Check sheet for the modelled part. Datum: model origin and axes. Units: mm. A direction names the side the tool comes from. Round coordinates to 2 decimals unless told otherwise and drop trailing zeros. Order: outer loops, then holes, each group sorted by start corner. A loop starts at its lowest first (then second) coordinate and runs counter-clockwise, first axis right, second up.
from build123d import *

# Parameters (mm, degrees)
BOSS_EXTRUDE1_DEPTH           = 4
BOSS_EXTRUDE1_DRAFT           = -2
SHELL1_T                      = -0.5
BOSS_EXTRUDE2_DEPTH           = 5.5
BOSS_EXTRUDE2_DRAFT           = 1.5
BOSS_EXTRUDE2_PROFILE_2_DEPTH = 5.5
BOSS_EXTRUDE2_PROFILE_2_DRAFT = 1.5
BOSS_EXTRUDE2_PROFILE_3_DEPTH = 5.5
BOSS_EXTRUDE2_PROFILE_3_DRAFT = 1.5
BOSS_EXTRUDE2_PROFILE_4_DEPTH = 5.5
BOSS_EXTRUDE2_PROFILE_4_DRAFT = 1.5


with BuildPart() as part:
    # Sketch1 → Boss-Extrude1 (with draft: the straight prism first)
    with BuildSketch(Plane(origin=(0, 0, 0), x_dir=(1, 0, 0), z_dir=(0, 1, 0))):
        with BuildLine():
            Line((-7.5, -6.375), (7.5, -6.375))
            ThreePointArc((7.5, -6.375), (8.207106781, -6.082106781), (8.5, -5.375))
            Line((8.5, -5.375), (8.5, 5.375))
            ThreePointArc((8.5, 5.375), (8.207106781, 6.082106781), (7.5, 6.375))
            Line((7.5, 6.375), (-7.5, 6.375))
            ThreePointArc((-7.5, 6.375), (-8.207106781, 6.082106781), (-8.5, 5.375))
            Line((-8.5, 5.375), (-8.5, -5.375))
            ThreePointArc((-8.5, -5.375), (-8.207106781, -6.082106781), (-7.5, -6.375))
        make_face()
    extrude(amount=-BOSS_EXTRUDE1_DEPTH)
    # Boss-Extrude1: the draft: its side faces are tilted about the plane it starts from
    boss_extrude1_sides = [part.faces().sort_by_distance(p)[0] for p in [
        (0, -2, 6.375),
        (8.207106781, -2, 6.082106781),
        (8.5, -2, 0),
        (8.207106781, -2, -6.082106781),
        (0, -2, -6.375),
        (-8.207106781, -2, -6.082106781),
        (-8.5, -2, 0),
        (-8.207106781, -2, 6.082106781),
    ]]
    draft(boss_extrude1_sides, Plane(origin=(0, 0, 0), x_dir=(1, 0, 0), z_dir=(0, 1, 0)), BOSS_EXTRUDE1_DRAFT)

    # Shell1
    shell1_openings = [part.faces().sort_by_distance(p)[0] for p in [
        (0, 0, 0),
    ]]
    offset(amount=SHELL1_T, openings=shell1_openings, kind=Kind.INTERSECTION)


with BuildPart() as boss_extrude2_tool:
    # Sketch3 → Boss-Extrude2 (with draft: the straight prism first)
    with BuildSketch(Plane(origin=(0, -3.5, 0), x_dir=(1, 0, 0), z_dir=(0, 1, 0))):
        with BuildLine():
            ThreePointArc((-0.6, 2.897704648), (-2.092449787, 2.092449787), (-2.897704648, 0.6))
            Line((-2.897704648, 0.6), (-0.6, 0.6))
            Line((-0.6, 0.6), (-0.6, 2.897704648))
        make_face()
    extrude(amount=BOSS_EXTRUDE2_DEPTH)
    # Boss-Extrude2: the draft: its side faces are tilted about the plane it starts from
    boss_extrude2_sides = [boss_extrude2_tool.faces().sort_by_distance(p)[0] for p in [
        (-2.092449787, -0.75, -2.092449787),
        (-1.748852324, -0.75, -0.6),
        (-0.6, -0.75, -1.748852324),
    ]]
    draft(boss_extrude2_sides, Plane(origin=(0, -3.5, 0), x_dir=(1, 0, 0), z_dir=(0, 1, 0)), BOSS_EXTRUDE2_DRAFT)


with BuildPart() as part_1:
    add(part.part)

    # Boss-Extrude2: add boss_extrude2_tool
    add(boss_extrude2_tool.part)


with BuildPart() as boss_extrude2_profile_2_tool:
    # Sketch3 → Boss-Extrude2 profile 2 (with draft: the straight prism first)
    with BuildSketch(Plane(origin=(0, -3.5, 0), x_dir=(1, 0, 0), z_dir=(0, 1, 0))):
        with BuildLine():
            Line((0.6, 2.897704648), (0.6, 0.6))
            Line((0.6, 0.6), (2.897704648, 0.6))
            ThreePointArc((2.897704648, 0.6), (2.092449787, 2.092449787), (0.6, 2.897704648))
        make_face()
    extrude(amount=BOSS_EXTRUDE2_PROFILE_2_DEPTH)
    # Boss-Extrude2 profile 2: the draft: its side faces are tilted about the plane it starts from
    boss_extrude2_profile_2_sides = [boss_extrude2_profile_2_tool.faces().sort_by_distance(p)[0] for p in [
        (2.092449787, -0.75, -2.092449787),
        (0.6, -0.75, -1.748852324),
        (1.748852324, -0.75, -0.6),
    ]]
    draft(boss_extrude2_profile_2_sides, Plane(origin=(0, -3.5, 0), x_dir=(1, 0, 0), z_dir=(0, 1, 0)), BOSS_EXTRUDE2_PROFILE_2_DRAFT)


with BuildPart() as part_2:
    add(part_1.part)

    # Boss-Extrude2 profile 2: add boss_extrude2_profile_2_tool
    add(boss_extrude2_profile_2_tool.part)


with BuildPart() as boss_extrude2_profile_3_tool:
    # Sketch3 → Boss-Extrude2 profile 3 (with draft: the straight prism first)
    with BuildSketch(Plane(origin=(0, -3.5, 0), x_dir=(1, 0, 0), z_dir=(0, 1, 0))):
        with BuildLine():
            ThreePointArc((-2.897704648, -0.6), (-2.092449787, -2.092449787), (-0.6, -2.897704648))
            Line((-0.6, -2.897704648), (-0.6, -0.6))
            Line((-0.6, -0.6), (-2.897704648, -0.6))
        make_face()
    extrude(amount=BOSS_EXTRUDE2_PROFILE_3_DEPTH)
    # Boss-Extrude2 profile 3: the draft: its side faces are tilted about the plane it starts from
    boss_extrude2_profile_3_sides = [boss_extrude2_profile_3_tool.faces().sort_by_distance(p)[0] for p in [
        (-2.092449787, -0.75, 2.092449787),
        (-0.6, -0.75, 1.748852324),
        (-1.748852324, -0.75, 0.6),
    ]]
    draft(boss_extrude2_profile_3_sides, Plane(origin=(0, -3.5, 0), x_dir=(1, 0, 0), z_dir=(0, 1, 0)), BOSS_EXTRUDE2_PROFILE_3_DRAFT)


with BuildPart() as part_3:
    add(part_2.part)

    # Boss-Extrude2 profile 3: add boss_extrude2_profile_3_tool
    add(boss_extrude2_profile_3_tool.part)


with BuildPart() as boss_extrude2_profile_4_tool:
    # Sketch3 → Boss-Extrude2 profile 4 (with draft: the straight prism first)
    with BuildSketch(Plane(origin=(0, -3.5, 0), x_dir=(1, 0, 0), z_dir=(0, 1, 0))):
        with BuildLine():
            Line((0.6, -0.6), (0.6, -2.897704648))
            ThreePointArc((0.6, -2.897704648), (2.092449787, -2.092449787), (2.897704648, -0.6))
            Line((2.897704648, -0.6), (0.6, -0.6))
        make_face()
    extrude(amount=BOSS_EXTRUDE2_PROFILE_4_DEPTH)
    # Boss-Extrude2 profile 4: the draft: its side faces are tilted about the plane it starts from
    boss_extrude2_profile_4_sides = [boss_extrude2_profile_4_tool.faces().sort_by_distance(p)[0] for p in [
        (1.748852324, -0.75, 0.6),
        (0.6, -0.75, 1.748852324),
        (2.092449787, -0.75, 2.092449787),
    ]]
    draft(boss_extrude2_profile_4_sides, Plane(origin=(0, -3.5, 0), x_dir=(1, 0, 0), z_dir=(0, 1, 0)), BOSS_EXTRUDE2_PROFILE_4_DRAFT)


with BuildPart() as part_4:
    add(part_3.part)

    # Boss-Extrude2 profile 4: add boss_extrude2_profile_4_tool
    add(boss_extrude2_profile_4_tool.part)


solid = part_4.part
1) Sectioned sample at B-B on z = 5. Record the cut outline in (x, y).
2) Sectioned sample at A-A on y = -3.25. Record the cut outline in (x, z) (1 decimal).
3) Draft check along Z on faces 3 (the face through (0, -3.5, 0)), 4 (the face through (-2, 2, 1)), 5 (the face through (-8.166, -1.972, 6.026)), 6 (the face through (-2.059, -0.788, 2.026)). Enter one of: pulls with the +Z half, pulls with the -Z half, needs draft (parallel to the pull), parting line crosses it, or undercut.
4) Set-up check for faces 1 (the face through (2.059, -0.788, -2.026)), 2 (the face through (-1.5, 2, -1.5)): record each of +Z, -Z, +X, -X, +Y, -Y from which the full face is reachable in a straight line by a thin tool's end or side.
5) Sectioned sample at D-D on y = -2.3. Record the cut outline in (x, z) (1 decimal).
6) Sectioned sample at C-C on x = -7. Record the cut outline in (y, z) (3 decimals), and give its area (3 significant figures).
7) Scan lines: line 1 (X direction, y = -1.6, z = -2); line 2 (X direction, y = -2.4, z = 2.25); line 3 (Y direction, x = -4.75, z = -2). Record each from-to range of solid material in increasing order.
8) Gauge pin test, flat ends, axial feed: pin 1 (6 mm diameter, centred on x = 6, z = 4.5, fed in from +Y); pin 2 (1 mm diameter, centred on x = -6.5, z = -1.5, fed in from +Y); pin 3 (1.5 mm diameter, centred on x = 1, y = -2.5, fed in from -Z). Record the tip position at first contact, or that the pin passes through.
Values found:
1. outline: (-8.5, 0) - (-8.36, -4) - (8.36, -4) - (8.5, 0) - (8, 0) - (7.88, -3.5) - (-7.88, -3.5) - (-8, 0) - close
2. outline: (-8.4, -5.4) arc R0.9 ccw to (-7.5, -6.3) - (7.5, -6.3) arc R0.9 ccw to (8.4, -5.4) - (8.4, 5.4) arc R0.9 ccw to (7.5, 6.3) - (-7.5, 6.3) arc R0.9 ccw to (-8.4, 5.4) - close; (-2.9, -0.6) arc R3 ccw to (-0.6, -2.9) - (-0.6, -0.6) - close; (-2.9, 0.6) - (-0.6, 0.6) - (-0.6, 2.9) arc R3 ccw to start; (0.6, -2.9) arc R3 ccw to (2.9, -0.6) - (0.6, -0.6) - close; (0.6, 0.6) - (2.9, 0.6) arc R3 ccw to (0.6, 2.9) - close; hole (-7.9, -5.4) arc R0.4 ccw to (-7.5, -5.8) - (7.5, -5.8) arc R0.4 ccw to (7.9, -5.4) - (7.9, 5.4) arc R0.4 ccw to (7.5, 5.8) - (-7.5, 5.8) arc R0.4 ccw to (-7.9, 5.4) - close
3. face 3: undercut
3. face 4: needs draft
3. face 5: pulls with the +Z half
3. face 6: undercut
4. face 1: +Y
4. face 2: +Z, -Z, +X, -X, +Y
5. outline: (-8.4, -5.4) arc R0.9 ccw to (-7.5, -6.3) - (7.5, -6.3) arc R0.9 ccw to (8.4, -5.4) - (8.4, 5.4) arc R0.9 ccw to (7.5, 6.3) - (-7.5, 6.3) arc R0.9 ccw to (-8.4, 5.4) - close; (-2.9, -0.6) arc R2.9 ccw to (-0.6, -2.9) - (-0.6, -0.6) - close; (-2.9, 0.6) - (-0.6, 0.6) - (-0.6, 2.9) arc R2.9 ccw to start; (0.6, -2.9) arc R2.9 ccw to (2.9, -0.6) - (0.6, -0.6) - close; (0.6, 0.6) - (2.9, 0.6) arc R2.9 ccw to (0.6, 2.9) - close; hole (-7.9, -5.4) arc R0.4 ccw to (-7.5, -5.8) - (7.5, -5.8) arc R0.4 ccw to (7.9, -5.4) - (7.9, 5.4) arc R0.4 ccw to (7.5, 5.8) - (-7.5, 5.8) arc R0.4 ccw to (-7.9, 5.4) - close
6. outline: (-4, -6.235) - (0, -6.375) - (0, -5.875) - (-3.5, -5.752) - (-3.5, 5.752) - (0, 5.875) - (0, 6.375) - (-4, 6.235) - close
6. area: 9.75 mm2
7. line 1: x = -8.44 to -7.94, -2.11 to -0.65, 0.65 to 2.11, 7.94 to 8.44
7. line 2: x = -8.42 to -7.92, -1.88 to -0.63, 0.63 to 1.88, 7.92 to 8.42
7. line 3: y = -4 to -3.5
8. pin 1: stops at y = 0
8. pin 2: stops at y = -3.5
8. pin 3: stops at z = -6.31
